Can you work these out from the drawing? Everything is in mm from the part's minimum corner. Give positions to 0.01 mm unless a question says otherwise; leave off trailing zeros. Order: outer loops, then holes, each group sorted by start corner. A loop starts at its lowest first (then second) coordinate and runs counter-clockwise, first axis right, second up. Notation, with made-up numbers: (25, 62.5) - (68, 62.5) arc R24 cw to (68, 93.5) - close; hole circle Ø7 at (74, 66). An arc over 180 degrees is marked (long way). Answer as a JSON object with one key per item and string values.
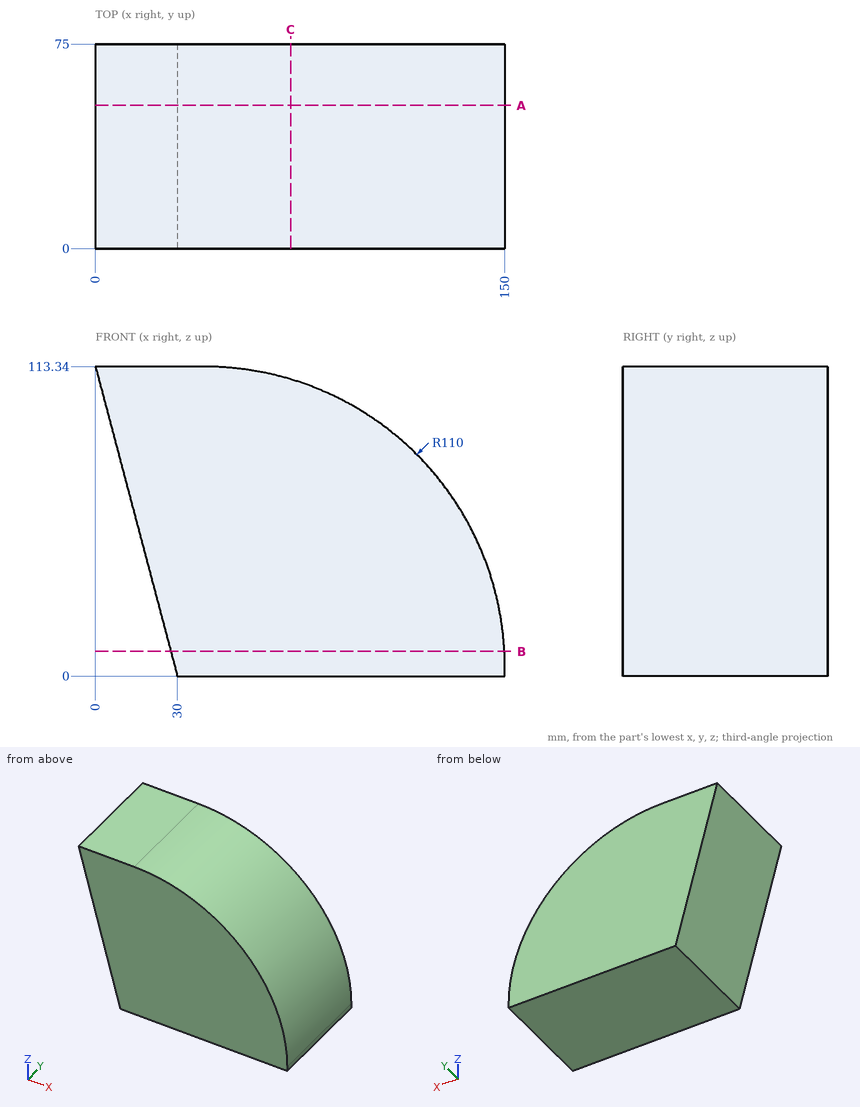
Q1. I need wall thicknesses on L1, parallel to Z at x = 47, y = 18; L2, parallel to X at y = 43, z = 87.5; L3, parallel to X at y = 64, z = 64. Which ranges of each line are inside material? Lowest first, please.
Recorded:
{"L1": "z = 0 to 113.12", "L2": "x = 6.84 to 110.83", "L3": "x = 13.06 to 131.76"}
Q2. If we section it at C-C, the plane x = 71.5: Please give me the cut outline in (y, z).
Recorded:
{"outline": "(0, 0) - (75, 0) - (75, 108.73) - (0, 108.73) - close"}
Q3. If we section it at B-B, the plane z = 9: Please give me the cut outline in (x, y).
Recorded:
{"outline": "(27.62, 0) - (149.85, 0) - (149.85, 75) - (27.62, 75) - close"}
Q4. I'm going to push flat-ended pins straight in: pin 1 Ø10 at (x, y) = (44.5, 47) entering from -Z; pin 2 Ø12 at (y, z) = (55, 91) entering from +X; pin 3 Ø5 at (x, y) = (61.5, 27) entering from +Z. Where does each tip first touch, or does it pass through?
Recorded:
{"pin 1": "stops at z = 0", "pin 2": "stops at x = 113.7", "pin 3": "stops at z = 111.69"}
Q5. If we section it at A-A, the plane y = 52.5: Please give me the cut outline in (x, z), then the cut area to 3 significant figures.
Recorded:
{"outline": "(0, 113.34) - (30, 0) - (150, 0) - (150, 3.34) arc R110 ccw to (40, 113.34) - close", "area": "12,700 mm^2"}
